from build123d import *

# Parameters (mm, degrees)
SKETCH_1_W          = 31
SKETCH_1_H          = 26.5
EXTRUDE_1_DEPTH     = 20
SKETCH_3_W          = 16
SKETCH_3_H          = 16
CUT_EXTRUDE_1_DEPTH = 23.5
SKETCH_4_W          = 6.1
SKETCH_4_H          = 6.2
EXTRUDE_2_DEPTH     = 4
SKETCH_5_W          = 6.2
SKETCH_5_H          = 6.1
EXTRUDE_3_DEPTH     = 2
SKETCH_6_R          = 3.2
CUT_EXTRUDE_2_DEPTH = 37.640141921
CUT_EXTRUDE_3_DEPTH = 31.623724463
SKETCH_9_W          = 2.5
SKETCH_9_H          = 5.6
CUT_EXTRUDE_4_DEPTH = 8.3
SKETCH_10_W         = 1
SKETCH_10_H         = 15.952878331
CUT_EXTRUDE_5_DEPTH = 1.72
SKETCH_11_R         = 5.5
CUT_EXTRUDE_6_DEPTH = 11
SKETCH_12_R         = 2.05
CUT_EXTRUDE_7_DEPTH = 40.629534441
CUT_EXTRUDE_8_REACH = 42.725
FILLET_2_R          = 1
FILLET_3_R          = 1
SKETCH_14_R         = 1.6
CUT_EXTRUDE_9_DEPTH = 2.25
CHAMFER_2_SIZE      = 0.4
EXTRUDE_START       = 0.2
EXTRUDE_4_DEPTH     = 0.2
EXTRUDE_START_2     = 0.4
SKETCH_15_4_W       = 0.7
SKETCH_15_4_H       = 6.4
EXTRUDE_5_DEPTH     = 0.4
FILLET_4_R          = 2
FILLET_5_R          = 0.4
CHAMFER_3_SIZE      = 0.4
CHAMFER_4_SIZE      = 0.4
CHAMFER_5_SIZE      = 1


with BuildPart() as part:
    # 草图1 → 凸台-拉伸1 (new body)
    with BuildSketch(Plane.XY):
        Rectangle(SKETCH_1_W, SKETCH_1_H)
    extrude(amount=EXTRUDE_1_DEPTH)

    # 草图3 → 切除-拉伸1 (cut)
    with BuildSketch(Plane(origin=(0, 13.25, 0), x_dir=(1, 0, 0), z_dir=(0, 1, 0))):
        with Locations((6.5, -10.108217082)):
            Rectangle(SKETCH_3_W, SKETCH_3_H)
    extrude(amount=-CUT_EXTRUDE_1_DEPTH, mode=Mode.SUBTRACT)

    # 草图4 → 凸台-拉伸2 (add)
    with BuildSketch(Plane(origin=(0, 13.25, 0), x_dir=(1, 0, 0), z_dir=(0, 1, 0))):
        with Locations((-12.45, -9.9)):
            Rectangle(SKETCH_4_W, SKETCH_4_H)
    extrude(amount=EXTRUDE_2_DEPTH)

    # 草图5 → 凸台-拉伸3 (add)
    with BuildSketch(Plane(origin=(0, 13.25, 0), x_dir=(1, 0, 0), z_dir=(0, 1, 0))):
        with Locations((-5.5, -3.05)):
            Rectangle(SKETCH_5_W, SKETCH_5_H)
        with Locations((-5.5, -16.95)):
            Rectangle(SKETCH_5_W, SKETCH_5_H)
    extrude(amount=EXTRUDE_3_DEPTH)

    # 草图6 → 切除-拉伸2 (cut, through all)
    with BuildSketch(Plane(origin=(0, 13.25, 0), x_dir=(1, 0, 0), z_dir=(0, 1, 0))):
        with Locations(Location((-5.4, -10, 0), (0, 0, 270))):
            Circle(SKETCH_6_R)
    extrude(amount=-CUT_EXTRUDE_2_DEPTH, mode=Mode.SUBTRACT)

    # 草图8 → 切除-拉伸3 (cut, through all)
    with BuildSketch(Plane.XY.offset(20)):
        with BuildLine():
            Line((5.9, 10.65), (7.1, 10.65))
            ThreePointArc((7.1, 10.65), (8.514213562, 10.064213562), (9.1, 8.65))
            Line((9.1, 8.65), (9.1, 4.85))
            ThreePointArc((9.1, 4.85), (8.514213562, 3.435786438), (7.1, 2.85))
            Line((7.1, 2.85), (5.9, 2.85))
            ThreePointArc((5.9, 2.85), (4.485786438, 3.435786438), (3.9, 4.85))
            Line((3.9, 4.85), (3.9, 8.65))
            ThreePointArc((3.9, 8.65), (4.485786438, 10.064213562), (5.9, 10.65))
        make_face()
    extrude(amount=-CUT_EXTRUDE_3_DEPTH, mode=Mode.SUBTRACT)

    # 草图9 → 切除-拉伸4 (cut)
    with BuildSketch(Plane.XY.offset(20)):
        with Locations((-12, 7.25)):
            Rectangle(SKETCH_9_W, SKETCH_9_H)
        with Locations((-12, -2.75)):
            Rectangle(SKETCH_9_W, SKETCH_9_H)
    cut_extrude_4 = extrude(amount=-CUT_EXTRUDE_4_DEPTH, mode=Mode.SUBTRACT)

    # 草图10 → 切除-拉伸5 (cut)
    with BuildSketch(Plane(origin=(0, 13.25, 0), x_dir=(1, 0, 0), z_dir=(0, 1, 0))):
        with Locations((15, -10.084656247)):
            Rectangle(SKETCH_10_W, SKETCH_10_H)
    extrude(amount=-CUT_EXTRUDE_5_DEPTH, mode=Mode.SUBTRACT)

    # 草图11 → 切除-拉伸6 (cut)
    with BuildSketch(Plane.XZ.offset(13.25)):
        with Locations(Location((-5.5, 10, 0), (0, 0, 270))):
            Circle(SKETCH_11_R)
    extrude(amount=-CUT_EXTRUDE_6_DEPTH, mode=Mode.SUBTRACT)

    # 草图12 → 切除-拉伸7 (cut, through all)
    with BuildSketch(Plane(origin=(0, -13.25, 0), x_dir=(-1, 0, 0), z_dir=(0, -1, 0))):
        with Locations(Location((-7.5, -10, 0), (0, 0, 90))):
            Circle(SKETCH_12_R)
    extrude(amount=-CUT_EXTRUDE_7_DEPTH, mode=Mode.SUBTRACT)

    # 草图13 → 切除-拉伸8 (cut, up to next)
    with BuildSketch(Plane(origin=(15.5, 0, 0), x_dir=(0, 0, -1), z_dir=(1, 0, 0)), mode=Mode.PRIVATE) as cut_extrude_8_sk1:
        with BuildLine():
            Line((-10.2, -4.7), (-9.8, -4.7))
            ThreePointArc((-9.8, -4.7), (-8.25, -6.25), (-9.8, -7.8))
            Line((-9.8, -7.8), (-10.2, -7.8))
            ThreePointArc((-10.2, -7.8), (-11.75, -6.25), (-10.2, -4.7))
        make_face()
    cut_extrude_8_tool1 = extrude(cut_extrude_8_sk1.sketch, amount=-CUT_EXTRUDE_8_REACH, mode=Mode.PRIVATE) & part.part
    add(cut_extrude_8_tool1.solids().sort_by_distance((15.5, -6.25, 10))[0], mode=Mode.SUBTRACT)

    # 圆角2
    fillet_2_edges = [part.edges().sort_by_distance(p)[0] for p in [
        (15.5, 0, 20),
        (-15.5, 0, 20),
        (15.5, 0, 0),
        (-15.5, 0, 0),
    ]]
    fillet(fillet_2_edges, radius=FILLET_2_R)

    # 圆角3
    # the kernel refuses this fillet: 1 mm, written as the material it takes off along each edge
    with BuildSketch(Plane(origin=(15.5, 15.745329826, 18.061095413), x_dir=(0, 0, 1), z_dir=(0, -1, 0))) as fillet_3_piece_1:
        with BuildLine():
            CenterArc((1, 0.99813193), FILLET_3_R, 180, 86.497309331)
            Line((0, 0.99813193), (-0.02, 0.99813193))
            Line((-0.02, 0.99813193), (-0.02, 0))
            Line((-0.02, 0), (0, -0.02))
            ThreePointArc((0, -0.02), (0.469452294, -0.02), (0.937682679, -0.019962639))
            Line((0.937682679, -0.019962639), (0.938904587, 0))
        make_face()
    extrude(amount=4.215329826, mode=Mode.SUBTRACT)
    with BuildSketch(Plane(origin=(15.5, 15.75, 2.108217082), x_dir=(0, 0, -1), z_dir=(0, -1, 0))) as fillet_3_piece_2:
        with BuildLine():
            CenterArc((FILLET_3_R, -FILLET_3_R), FILLET_3_R, 90, 90)
            Line((0, -FILLET_3_R), (-FILLET_3_R * 0.02, -FILLET_3_R))
            Line((-FILLET_3_R * 0.02, -FILLET_3_R), (-FILLET_3_R * 0.02, FILLET_3_R * 0.02))
            Line((-FILLET_3_R * 0.02, FILLET_3_R * 0.02), (FILLET_3_R, FILLET_3_R * 0.02))
            Line((FILLET_3_R, FILLET_3_R * 0.02), (FILLET_3_R, 0))
        make_face()
    extrude(amount=4.22, mode=Mode.SUBTRACT)

    # 草图14 → 切除-拉伸9 (cut)
    with BuildSketch(Plane.ZY.offset(15.5)):
        with Locations((5, 7.25)):
            Circle(SKETCH_14_R)
        with Locations((15, 7.25)):
            Circle(SKETCH_14_R)
        with Locations((5, -2.75)):
            Circle(SKETCH_14_R)
        with Locations((15, -2.75)):
            Circle(SKETCH_14_R)
    extrude(amount=-CUT_EXTRUDE_9_DEPTH, mode=Mode.SUBTRACT)

    # 镜向1: 切除-拉伸4 across plane
    add(cut_extrude_4.mirror(Plane(origin=(0, 0, 10), x_dir=(1, 0, 0), z_dir=(0, 0, -1))), mode=Mode.SUBTRACT)

    # 倒角2
    chamfer_2_edges = [part.edges().sort_by_distance(p)[0] for p in [
        (0, -13.25, 20),
        (0, -13.25, 0),
        (15.5, -13.25, 10),
        (-15.5, -13.25, 10),
        (15.207106781, -13.25, 0.292893219),
        (15.207106781, -13.25, 19.707106781),
        (-15.207106781, -13.25, 0.292893219),
        (-15.207106781, -13.25, 19.707106781),
    ]]
    chamfer(chamfer_2_edges, length=CHAMFER_2_SIZE)

    # 草图15 → 凸台-拉伸4 (add)
    with BuildSketch(Plane.XZ.offset(2.25).offset(EXTRUDE_START)):
        with BuildLine():
            Line((-8.6, 13.2), (-8.6, 14.543126677))
            ThreePointArc((-8.6, 14.543126677), (-9.3457172, 13.931979046), (-9.973253849, 13.2))
            Line((-9.973253849, 13.2), (-8.6, 13.2))
        make_face()
        with BuildLine():
            ThreePointArc((-2.2, 14.4), (-5.377031258, 15.498625163), (-8.6, 14.543126677))
            Line((-8.6, 14.543126677), (-8.6, 13.2))
            Line((-8.6, 13.2), (-2.2, 13.2))
            Line((-2.2, 13.2), (-2.2, 14.4))
        make_face()
        with BuildLine():
            ThreePointArc((-1.5, 13.774917218), (-1.836643326, 14.102416103), (-2.2, 14.4))
            Line((-2.2, 14.4), (-2.2, 13.2))
            Line((-2.2, 13.2), (-1.5, 13.2))
            Line((-1.5, 13.2), (-1.5, 13.774917218))
        make_face()
        with BuildLine():
            Line((-8.6, 5.456873323), (-8.6, 6.8))
            Line((-8.6, 6.8), (-9.973253849, 6.8))
            ThreePointArc((-9.973253849, 6.8), (-9.3457172, 6.068020954), (-8.6, 5.456873323))
        make_face()
        with BuildLine():
            Line((-2.2, 6.8), (-8.6, 6.8))
            Line((-8.6, 6.8), (-8.6, 5.456873323))
            ThreePointArc((-8.6, 5.456873323), (-5.377031258, 4.501374837), (-2.2, 5.6))
            Line((-2.2, 5.6), (-2.2, 6.8))
        make_face()
        with BuildLine():
            Line((-1.5, 6.8), (-2.2, 6.8))
            Line((-2.2, 6.8), (-2.2, 5.6))
            ThreePointArc((-2.2, 5.6), (-1.836643326, 5.897583897), (-1.5, 6.225082782))
            Line((-1.5, 6.225082782), (-1.5, 6.8))
        make_face()
    extrude(amount=-EXTRUDE_4_DEPTH)

    # 草图15<4> → 凸台-拉伸5 (add)
    with BuildSketch(Plane.XZ.offset(2.25).offset(EXTRUDE_START_2)):
        with BuildLine():
            Line((-8.6, 13.2), (-8.6, 14.543126677))
            ThreePointArc((-8.6, 14.543126677), (-9.3457172, 13.931979046), (-9.973253849, 13.2))
            Line((-9.973253849, 13.2), (-8.6, 13.2))
        make_face()
        with BuildLine():
            Line((-8.6, 6.8), (-8.6, 13.2))
            Line((-8.6, 13.2), (-9.973253849, 13.2))
            ThreePointArc((-9.973253849, 13.2), (-11, 10), (-9.973253849, 6.8))
            Line((-9.973253849, 6.8), (-8.6, 6.8))
        make_face()
        with BuildLine():
            Line((-8.6, 5.456873323), (-8.6, 6.8))
            Line((-8.6, 6.8), (-9.973253849, 6.8))
            ThreePointArc((-9.973253849, 6.8), (-9.3457172, 6.068020954), (-8.6, 5.456873323))
        make_face()
        with BuildLine():
            ThreePointArc((-1.5, 13.774917218), (-1.836643326, 14.102416103), (-2.2, 14.4))
            Line((-2.2, 14.4), (-2.2, 13.2))
            Line((-2.2, 13.2), (-1.5, 13.2))
            Line((-1.5, 13.2), (-1.5, 13.774917218))
        make_face()
        with Locations((-1.85, 10)):
            Rectangle(SKETCH_15_4_W, SKETCH_15_4_H)
        with BuildLine():
            Line((-1.5, 6.8), (-2.2, 6.8))
            Line((-2.2, 6.8), (-2.2, 5.6))
            ThreePointArc((-2.2, 5.6), (-1.836643326, 5.897583897), (-1.5, 6.225082782))
            Line((-1.5, 6.225082782), (-1.5, 6.8))
        make_face()
    extrude(amount=-EXTRUDE_5_DEPTH)

    # 圆角4
    fillet_4_edges = [part.edges().sort_by_distance(p)[0] for p in [
        (-9.4, 15.25, 13),
        (-9.4, 15.25, 6.8),
        (-2.4, 14.25, 6.1),
        (-8.6, 14.25, 6.1),
        (-2.4, 14.25, 13.9),
        (-8.6, 14.25, 13.9),
    ]]
    fillet(fillet_4_edges, radius=FILLET_4_R)

    # 圆角5
    fillet_5_edges = [part.edges().sort_by_distance(p)[0] for p in [
        (-15.5, 15.25, 6.8),
        (-15.5, 15.25, 13),
        (-2.4, 14.25, 0),
        (-8.6, 14.25, 0),
        (-2.4, 14.25, 20),
        (-8.6, 14.25, 20),
    ]]
    fillet(fillet_5_edges, radius=FILLET_5_R)

    # 倒角3
    chamfer_3_edges = [part.edges().sort_by_distance(p)[0] for p in [
        (-8.6, 15.25, 17.75),
        (-5.5, 15.25, 13.9),
        (-2.985786438, 15.25, 14.485786438),
        (-8.014213562, 15.25, 14.485786438),
        (-9.4, 17.25, 9.9),
        (-13.25, 17.25, 6.8),
        (-9.985786438, 17.25, 7.385786438),
        (-9.985786438, 17.25, 12.414213562),
        (-2.4, 15.25, 2.25),
        (-5.5, 15.25, 6.1),
        (-8.014213562, 15.25, 5.514213562),
        (-2.985786438, 15.25, 5.514213562),
        (-5.5, 15.25, 20),
        (-2.4, 15.25, 17.75),
        (-2.517157288, 15.25, 19.882842712),
        (-8.482842712, 15.25, 19.882842712),
        (-5.5, 15.25, 0),
        (-8.6, 15.25, 2.25),
        (-8.482842712, 15.25, 0.117157288),
        (-2.517157288, 15.25, 0.117157288),
        (-13.25, 17.25, 13),
        (-15.5, 17.25, 9.9),
        (-15.382842712, 17.25, 6.917157288),
        (-15.382842712, 17.25, 12.882842712),
    ]]
    chamfer(chamfer_3_edges, length=CHAMFER_3_SIZE)

    # 倒角4
    chamfer_4_edges = [part.edges().sort_by_distance(p)[0] for p in [
        (-5.5, -13.25, 15.5),
    ]]
    chamfer(chamfer_4_edges, length=CHAMFER_4_SIZE)

    # 倒角5
    chamfer_5_edges = [part.edges().sort_by_distance(p)[0] for p in [
        (7.5, -13.25, 12.05),
    ]]
    chamfer(chamfer_5_edges, length=CHAMFER_5_SIZE)


solid = part.part
Could you check a few things on this model? Use its own coordinates, in mm. A direction names the side the tool comes from. Give positions to 0.01 mm unless a question says otherwise; leave off trailing zeros. Loops run counter-clockwise (first coordinate to the right, second up) from the corner with the lowest first, then second, coordinate; pieces in that order, holes last. Notation, with made-up numbers: (46.25, 79) -> (50.25, 79) arc R20 cw to (50.25, 89) -> close; hole circle Ø8 at (12, 22). An arc over 180 degrees is marked (long way). Answer as CSV lines item,"result". Start each with the question number.
(1) I need wall thicknesses on probe 1 along Y at (x, z) = (-12, 5.75); probe 2 along Y at (x, z) = (-14.85, 5); probe 3 along X at (y, z) = (-0.5, 9.75). Which ranges of each line are inside material? Lowest first, please.
(2) I'm going to push flat-ended pins straight in: pin 1 Ø1.7 at (y, z) = (7, 3.5) entering from -X; pin 2 Ø2 at (x, z) = (-2, 16.5) entering from +Y; pin 3 Ø1.3 at (y, z) = (14.5, 17.5) entering from +X; pin 4 Ø0.6 at (y, z) = (7, 0.5) entering from +X. Where does each tip first touch, or does it pass through?
(3) Which directions (+Z, -Z, +X, -X, +Y, -Y) give clear straight access to the entire face, cutting with the end or side of a thin tool? Please do faces 4 (the flat face through (-8.6, 14, 2)), 5 (the cylindrical face through (-14, 6, 14)), 6 (the flat face through (-2.8, -2.25, 7.6)).
(4) We'd pull the mould along X, two halves only. Please class faces 1 (the cylindrical face through (15.01, -6.28, 11.75)), 2 (the conical face through (15.042, -13.092, 0.47)), 3 (the cylindrical face through (8.5, 10.08, 1.07)): released by +X, released by -X, zero draft, split by the parting line, or undercut.
(5) If we section it at A-A on x = 7.5: Write out the boundary of the cut face in (y, z), then the cut area to 3 significant figures.
Computed:
1,probe 1,"y = -13.25 to -5.55, 0.05 to 4.45, 10.05 to 13.25"
1,probe 2,"y = -13.25 to -4.35, -1.15 to 5.65, 8.85 to 13.25"
1,probe 3,"x = -15.5 to -8.59, -2.21 to -1.5, 14.5 to 15.5"
2,pin 1,"stops at x = -15.5"
2,pin 2,"stops at y = 15.25"
2,pin 3,"stops at x = -2.4"
2,pin 4,"stops at x = 15.48"
3,face 4,"+Z, -Z, -X, +Y"
3,face 5,"-X"
3,face 6,"-Y"
4,face 1,"zero draft"
4,face 2,"released by +X"
4,face 3,"undercut"
5,outline,"(-13.25, 0.4) -> (-12.85, 0) -> (2.89, 0) -> (2.89, 2.11) -> (-10.25, 2.11) -> (-10.25, 7.95) -> (-12.25, 7.95) -> (-13.25, 6.95) -> close; (-13.25, 13.05) -> (-12.25, 12.05) -> (-10.25, 12.05) -> (-10.25, 18.11) -> (2.89, 18.11) -> (2.89, 20) -> (-12.85, 20) -> (-13.25, 19.6) -> close; (10.61, 0) -> (13.25, 0) -> (13.25, 2.11) -> (10.61, 2.11) -> close; (10.61, 18.11) -> (13.25, 18.11) -> (13.25, 20) -> (10.61, 20) -> close"
5,area,"110 mm2"
